Check sheet for the modelled part. Datum: model origin and axes. Units: mm. Face numbers are marked on the shaded views. A direction names the side the tool comes from. Round coordinates to 2 decimals unless told otherwise and drop trailing zeros. Order: outer loops, then holes, each group sorted by start corner. A loop starts at its lowest first (then second) coordinate and runs counter-clockwise, first axis right, second up. Notation, with made-up numbers: M 14.5,-20 L 36.5,-20 A12 cw 36.5,-16 Z; hole C 58.25,35.5 d1. An arc over 180 degrees is marked long. One line per item, written item: value. Start each with the question number.
(1) Access from +Z, -Z, +X, -X, +Y, -Y to the whole of each face (thin tool, end or side, straight path). Record for the marked faces 1, 2 and 3.
(2) Depth check by flat-ended pin: pin 1 Ø0.8 at (x, z) = (-0.5, 0.5) entering from -Y; pin 2 Ø0.5 at (x, z) = (6.5, -0.5) entering from -Y; pin 3 Ø1.1 at (y, z) = (0, -0.5) entering from +X. Enter the tip coordinate at first touch or a pass-through.
(3) Cross-section at C-C, the plane y = 3.75. Enter the section's corners in (x, z), and give its area (3 significant figures).
(4) Thickness scan on L1, parallel to Y at x = 6.5, z = -0.2; L2, parallel to Z at x = -2.5, y = 2.5; L3, parallel to Y at x = -7, z = -0.6. Record the ranges inside material, lowest first.
(5) Cross-section at D-D, the plane x = 6.5. Enter the section's corners in (y, z), and give its area (3 significant figures).
(6) Cross-section at B-B, the plane x = -7. Enter the section's corners in (y, z).
(7) Cross-section at A-A, the plane z = -0.7. Enter the section's corners in (x, y).
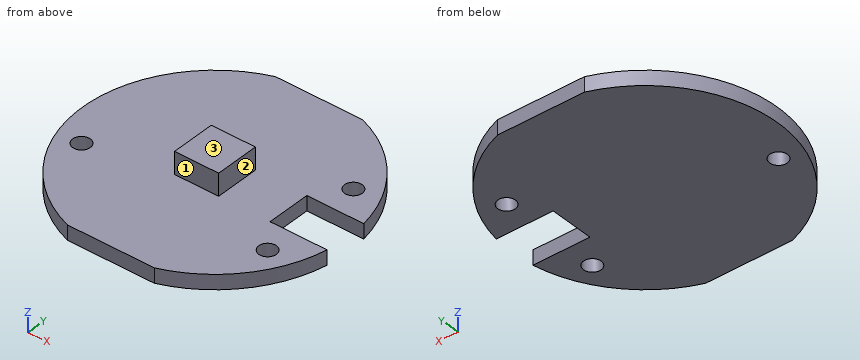
from build123d import *

# Parameters (mm, degrees)
SKETCH_1_R      = 0.6
EXTRUDE_1_DEPTH = 1
SKETCH_1_3_W    = 3
SKETCH_1_3_H    = 3
EXTRUDE_2_DEPTH = 1.5


with BuildPart() as part:
    # Sketch 1 → Extrude 1 (new body)
    with BuildSketch(Plane.XY):
        with BuildLine():
            Line((5, -1.5), (5, 1.5))
            Line((5, 1.5), (8.874119675, 1.5))
            ThreePointArc((8.874119675, 1.5), (6.873863542, 5.809475019), (2.958039892, 8.5))
            Line((2.958039892, 8.5), (-2.958039892, 8.5))
            ThreePointArc((-2.958039892, 8.5), (-9, 0), (-2.958039892, -8.5))
            Line((-2.958039892, -8.5), (2.958039892, -8.5))
            ThreePointArc((2.958039892, -8.5), (6.873863542, -5.809475019), (8.874119675, -1.5))
            Line((8.874119675, -1.5), (5, -1.5))
        make_face()
        with Locations((-7, -2.5)):
            Circle(SKETCH_1_R, mode=Mode.SUBTRACT)
        with Locations((6.5, -3.5)):
            Circle(SKETCH_1_R, mode=Mode.SUBTRACT)
        with Locations((6.5, 3.5)):
            Circle(SKETCH_1_R, mode=Mode.SUBTRACT)
    extrude(amount=-EXTRUDE_1_DEPTH)

    # Sketch 1_3 → Extrude 2 (add)
    with BuildSketch(Plane.XY):
        Rectangle(SKETCH_1_3_W, SKETCH_1_3_H)
    extrude(amount=EXTRUDE_2_DEPTH)


solid = part.part
Values found:
1. face 1: +Z, +X, -X, -Y
1. face 2: +Z, +X, +Y, -Y
1. face 3: +Z, +X, -X, +Y, -Y
2. pin 1: y = -1.5
2. pin 2: y = -6.48
2. pin 3: x = 5
3. outline: M -8.18,-1 L 5.95,-1 L 5.95,0 L -8.18,0 Z; M 7.05,-1 L 8.18,-1 L 8.18,0 L 7.05,0 Z
3. area: 15.3 mm^2
4. L1: -6.22 to -4.1, -2.9 to -1.5, 1.5 to 2.9, 4.1 to 6.22
4. L2: -1 to 0
4. L3: -5.66 to -3.1, -1.9 to 5.66
5. outline: M -6.22,-1 L -4.1,-1 L -4.1,0 L -6.22,0 Z; M -2.9,-1 L -1.5,-1 L -1.5,0 L -2.9,0 Z; M 1.5,-1 L 2.9,-1 L 2.9,0 L 1.5,0 Z; M 4.1,-1 L 6.22,-1 L 6.22,0 L 4.1,0 Z
5. area: 7.05 mm^2
6. outline: M -5.66,-1 L -3.1,-1 L -3.1,0 L -5.66,0 Z; M -1.9,-1 L 5.66,-1 L 5.66,0 L -1.9,0 Z
7. outline: M -2.96,-8.5 L 2.96,-8.5 A9 ccw 8.87,-1.5 L 5,-1.5 L 5,1.5 L 8.87,1.5 A9 ccw 2.96,8.5 L -2.96,8.5 A9 ccw Z; hole C -7,-2.5 d1.2; hole C 6.5,-3.5 d1.2; hole C 6.5,3.5 d1.2
